```python
from build123d import *

# Parameters (mm, degrees)
F1_DEPTH       = 150
F3_R           = 5
F4_DEPTH       = 12.5
F6_R           = 5
F7_DEPTH       = 12.5
F10_DEPTH      = 7.5
F10_DEPTH_BACK = 7.5
F13_R          = 10
F15_DEPTH      = 400
F15_DEPTH_BACK = 200
F18_DEPTH      = 190
F19_R          = 8


with BuildPart() as f1:
    # F0 (on Right) → F1 (new body)
    with BuildSketch(Plane.YZ):
        Polygon((45, 10), (0, 10), (-45, 10), (-45, -10), (45, -10), align=None)
    extrude(amount=F1_DEPTH)

    # F3 (on offset) → F4 (join)
    with BuildSketch(Plane.XZ.offset(45)):
        with BuildLine():
            Line((87.5, 10), (87.5, 20))
            ThreePointArc((87.5, 20), (75, 32.5), (62.5, 20))
            Line((62.5, 20), (62.5, 10))
            Line((62.5, 10), (75, 10))
            Line((75, 10), (87.5, 10))
        make_face()
        with Locations((75, 20)):
            Circle(F3_R, mode=Mode.SUBTRACT)
    extrude(amount=-F4_DEPTH)

    # F6 (on offset) → F7 (join)
    with BuildSketch(Plane(origin=(0, 45, 0), x_dir=(-1, 0, 0), z_dir=(0, 1, 0))):
        with BuildLine():
            Line((-62.5, 10), (-62.5, 20))
            ThreePointArc((-62.5, 20), (-75, 32.5), (-87.5, 20))
            Line((-87.5, 20), (-87.5, 10))
            Line((-87.5, 10), (-75, 10))
            Line((-75, 10), (-62.5, 10))
        make_face()
        with Locations((-75, 20)):
            Circle(F6_R, mode=Mode.SUBTRACT)
    extrude(amount=-F7_DEPTH)

    # F9 (on offset) → F10 (join, two sides)
    with BuildSketch(Plane(origin=(0, 0, 0), x_dir=(-1, 0, 0), z_dir=(0, 1, 0))) as f10_sk:
        with BuildLine():
            Line((-15, 10), (-15, 30))
            ThreePointArc((-15, 30), (-75, 90), (-135, 30))
            Line((-135, 30), (-135, 10))
            Line((-135, 10), (-75, 10))
            Line((-75, 10), (-15, 10))
        make_face()
    extrude(amount=F10_DEPTH)
    extrude(f10_sk.sketch, amount=-F10_DEPTH_BACK)

    # F14: sweep along a path in F11
    with BuildLine(Plane(origin=(0, 0, 0), x_dir=(-1, 0, 0), z_dir=(0, 1, 0))) as f14_path:
        Line((0, 0), (150, 0))
        Line((150, 0), (310.6493984302, -193.3859714218))
    # F13 (on offset) → F14 (sweep)
    with BuildSketch(Plane(origin=(0, 0, 0), x_dir=(0, -1, 0), z_dir=(-1, 0, 0))):
        Circle(F13_R)
    sweep(path=f14_path.line, transition=Transition.RIGHT)

    # F11 (on offset) → F15 (join, two sides)
    with BuildSketch(Plane(origin=(0, 0, 0), x_dir=(-1, 0, 0), z_dir=(0, 1, 0))) as f15_sk:
        Polygon((310.6493984302, -193.3859714218), (-375, -190), (-375, -210), (1649.8449922529, -221.7384290839), (1649.9710142492, -200), align=None)
    extrude(amount=F15_DEPTH)
    extrude(f15_sk.sketch, amount=-F15_DEPTH_BACK)

    # F17 (on offset) → F18 (join)
    with BuildSketch(Plane(origin=(0, 0, -10), x_dir=(1, 0, 0), z_dir=(0, 0, -1))):
        with BuildLine():
            ThreePointArc((65, 0), (75, -10), (85, 0))
            ThreePointArc((85, 0), (75, 10), (65, 0))
        make_face()
    extrude(amount=F18_DEPTH)

    # F19
    f19_edges = [f1.edges().sort_by_distance(p)[0] for p in [
        (0, -45, 0),
        (150, -45, 0),
        (150, 45, 0),
        (0, 45, 0),
    ]]
    fillet(f19_edges, radius=F19_R)


solid = f1.part
```
Source: CAD feature listing. Evaluate the final solid. Frame: model axes, mm. A direction names the side the tool comes from. Round coordinates to 2 decimals unless told otherwise and drop trailing zeros. Loops run counter-clockwise (first coordinate to the right, second up) from the corner with the lowest first, then second, coordinate; pieces in that order, holes last.
(1) Pull-direction query (Z, two-part tool) for faces 3 (the flat face through (74, 45, 2)), 4 (the cylindrical face through (73.681, 0.105, 89.985)), 5 (the flat face through (74, -11, -10)); classes: +Z half, -Z half, draft (parallel to the pull), parting line (faces both ways), or undercut.
From the geometry:
face 3: draft
face 4: +Z half
face 5: undercut
(2) Section query C-C (x = -868). Output: boundary loops of the cut face in (y, z), and give its area (3 significant figures).
From the geometry:
outline: (-200, -217.21) - (400, -217.21) - (400, -196.14) - (-200, -196.14) - close
area: 12,600 mm2
(3) Section query B-B (y = 139). Output: boundary loops of the cut face in (x, z) (3 decimals).
From the geometry:
outline: (-1649.971, -200) - (-1649.845, -221.738) - (375, -210) - (375, -190) - close
(4) Access query for faces 1 (the cylindrical face through (-222.46, 2.17, -102.5)), 2 (the flat face through (74, -45, 2)). Directions: +Z, -Z, +X, -X, +Y, -Y. A direction counts if a zero-diameter tool reaches every point of the face in a straight line with its end or side. Return the directions, or none.
From the geometry:
face 1: none
face 2: +Z, +X, -X, -Y
(5) Material intervals for probe 1 along Z at (x, y) = (75, -40); probe 2 along X at (y, z) = (21, 8.5); probe 3 along Y at (x, z) = (-68.5, -2.5), sorted ascending.
From the geometry:
probe 1: z = -211.74 to -191.48, -10 to 15, 25 to 32.5
probe 2: x = 0 to 150
probe 3: y = -9.68 to 9.68
(6) Contact query for flat-ended pins moving along their axis: pin 1 Ø16 at (y, z) = (-19.5, 4.5) entering from -X; pin 2 Ø8 at (y, z) = (-36, 15) entering from -X; pin 3 Ø8 at (y, z) = (-39.5, 17.5) entering from +X. Output: stop coordinate, or through.
From the geometry:
pin 1: stops at x = 0
pin 2: stops at x = 62.5
pin 3: stops at x = 87.5
(7) Section query A-A (x = -63.5). Output: boundary loops of the cut face in (y, z), and give its area (3 significant figures).
From the geometry:
outline: (-200, -212.54) - (400, -212.54) - (400, -192.17) - (-200, -192.17) - close; circle Ø20 at (0, 0)
area: 12,500 mm2
